Part print with two shaded views. Sizes in mm from the minimum x, y, z corner. A direction names the side the tool comes from. Round coordinates to 2 decimals unless told otherwise and drop trailing zeros. Write each loop counter-clockwise with the first axis right and the second up, starting at its lowest first coordinate (ties: lowest second). Pieces come first, ordered by that corner, then holes. Notation, with made-up numbers: (66.5, 55.25) -> (108.5, 55.25) arc R16 cw to (108.5, 73.25) -> close; hole circle Ø4 at (57, 20). An arc over 180 degrees is marked (long way). Put each result on its own line as item: value. Start each with the question number.
1. Saw through at C-C on x = 14.5. List the corners of the cut face in (y, z).
2. Saw through at A-A on y = 14.5. List the corners of the cut face in (x, z).
3. Drill centre lines: line 1 (Z direction, x = 24, y = 2); line 2 (Y direction, x = 34.5, z = 1.55); line 3 (Z direction, x = 23.5, y = 12.5). Where is each one in solid material? Low to high. Write a range as from..to.
4. 3-axis set-ups, long thin cutter, end or side, ignore diameter. For the marked faces 1 and 2: which of +Z, -Z, +X, -X, +Y, -Y reach the whole face in a straight line?
5. Saw through at B-B on z = 17. List the corners of the cut face in (x, y), and give its area (3 significant figures).
6. Flat gauge pins, fed straight in: P1, Ø8, axis at x = 9, z = 25.5, coming from the -Y side; P2, Ø10, axis at x = 30, y = 10, coming from the +Z side; P3, Ø3, axis at x = 11, z = 9.5, coming from the +Y side; P4, Ø8, axis at y = 10.5, z = 17, coming from the +X side. Where does each tip first touch, or does it go through?
7. Saw through at D-D on x = 20.5. List the corners of the cut face in (y, z).
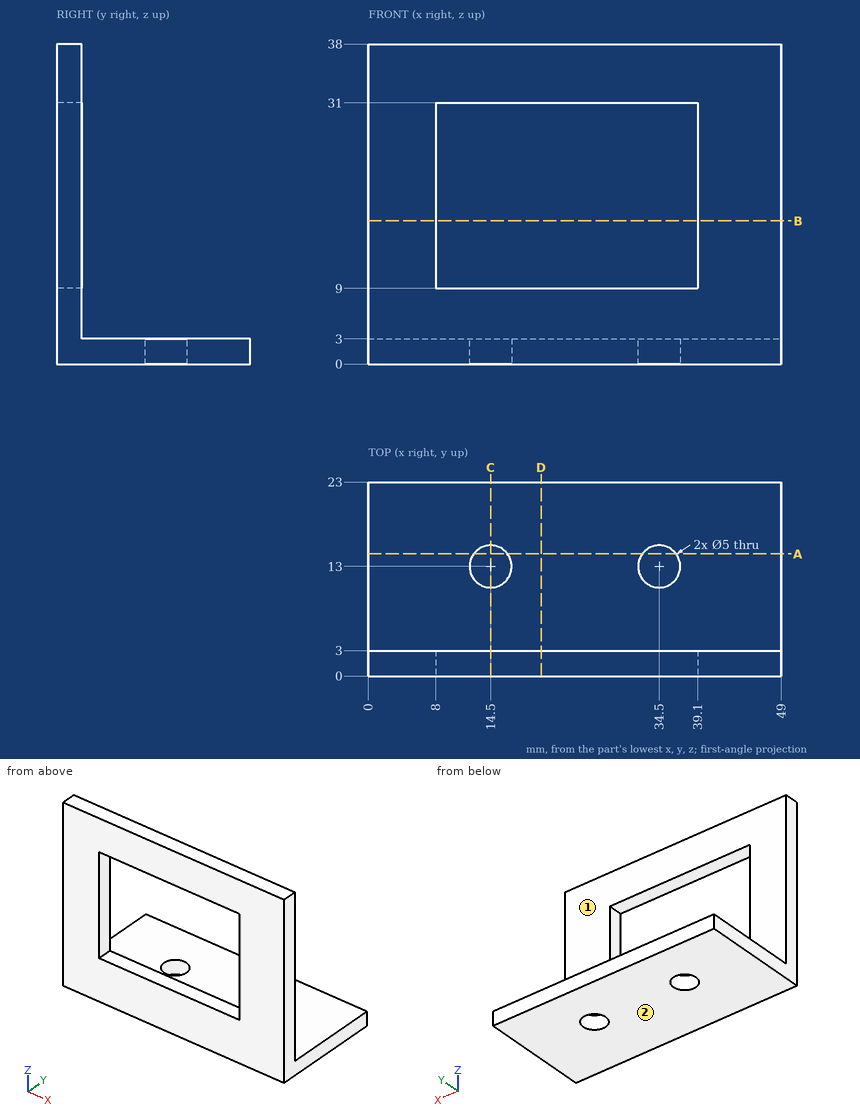
Return value:
1. outline: (0, 0) -> (10.5, 0) -> (10.5, 3) -> (3, 3) -> (3, 9) -> (0, 9) -> close; (0, 31) -> (3, 31) -> (3, 38) -> (0, 38) -> close; (15.5, 0) -> (23, 0) -> (23, 3) -> (15.5, 3) -> close
2. outline: (0, 0) -> (12.5, 0) -> (12.5, 3) -> (0, 3) -> close; (16.5, 0) -> (32.5, 0) -> (32.5, 3) -> (16.5, 3) -> close; (36.5, 0) -> (49, 0) -> (49, 3) -> (36.5, 3) -> close
3. line 1: z = 0..9, 31..38
3. line 2: y = 0..10.5, 15.5..23
3. line 3: z = 0..3
4. face 1: +Z, +X, -X, +Y
4. face 2: -Z, +X, -X, +Y, -Y
5. outline: (0, 0) -> (8, 0) -> (8, 3) -> (0, 3) -> close; (39.1, 0) -> (49, 0) -> (49, 3) -> (39.1, 3) -> close
5. area: 53.7 mm^2
6. P1: stops at y = 0
6. P2: stops at z = 3
6. P3: stops at y = 3
6. P4: passes through
7. outline: (0, 0) -> (23, 0) -> (23, 3) -> (3, 3) -> (3, 9) -> (0, 9) -> close; (0, 31) -> (3, 31) -> (3, 38) -> (0, 38) -> close
